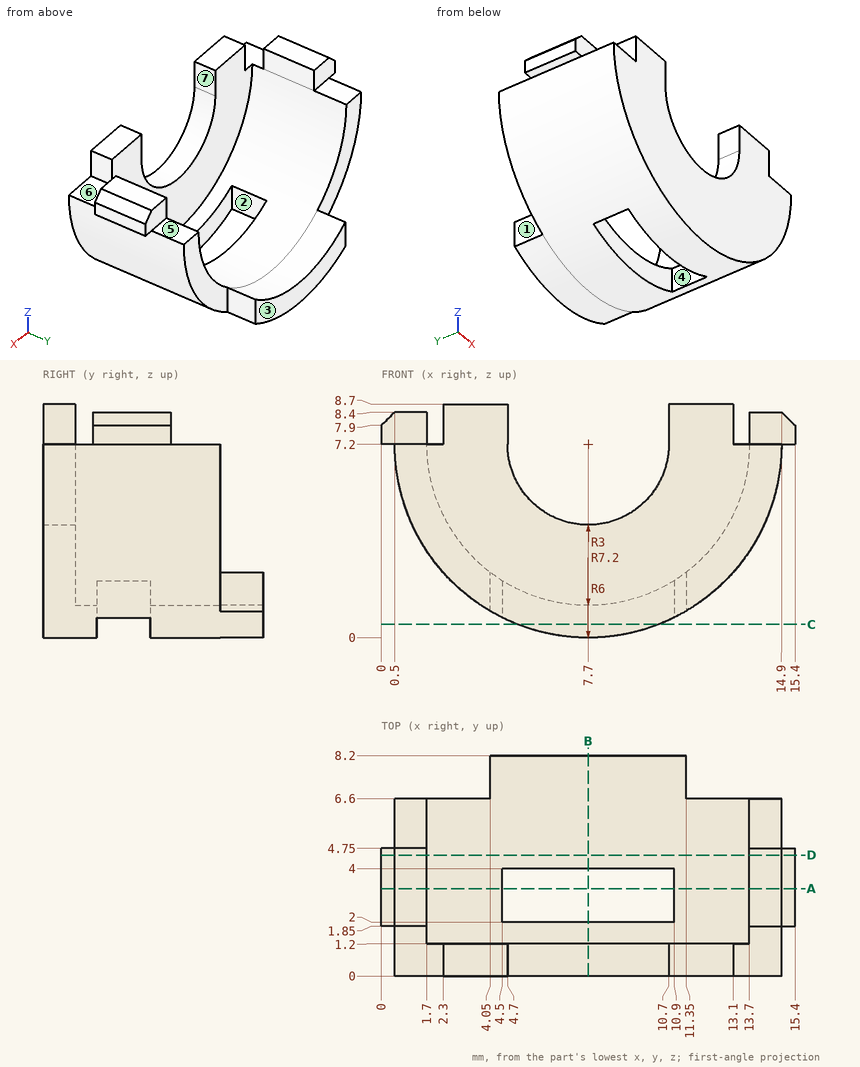
Geometry check sheet. Reference: drawing and pictorial views, mm from the part's lowest x, y, z. A direction names the side the tool comes from. Round coordinates to 2 decimals unless told otherwise and drop trailing zeros. Loops run counter-clockwise (first coordinate to the right, second up) from the corner with the lowest first, then second, coordinate; pieces in that order, holes last. Notation, with made-up numbers: M -37,6.5 L -31,6.5 A28 cw -31,36.5 Z; hole C 0.5,-1 d10. An arc over 180 degrees is marked long. One line per item, written item: value.
(1) Sectioned sample at B-B, the plane x = 7.7. Record the cut outline in (y, z), then the cut area to 3 significant figures.
Computed values:
outline: M 0,0 L 2,0 L 2,1.2 L 1.2,1.2 L 1.2,4.2 L 0,4.2 Z; M 4,0 L 8.2,0 L 8.2,1.2 L 4,1.2 Z
area: 11.0 mm^2
(2) Depth check by flat-ended pin: pin 1 Ø0.6 at (x, z) = (14.5, 8) entering from -Y; pin 2 Ø1 at (x, z) = (11, 3) entering from -Y; pin 3 Ø1 at (y, z) = (0.5, 7.5) entering from +X; pin 4 Ø4 at (y, z) = (7, 2) entering from +X. Enter the tip coordinate at first touch or a pass-through.
Computed values:
pin 1: stops at y = 1.85
pin 2: stops at y = 0
pin 3: stops at x = 14.9
pin 4: stops at x = 14.13
(3) Sectioned sample at A-A, the plane y = 3.25. Record the cut outline in (x, z).
Computed values:
outline: M 0,7.2 L 0.5,7.2 A7.2 ccw 4.5,0.75 L 4.5,2.12 A6 cw 1.7,7.2 L 1.7,8.4 L 0.5,8.4 L 0,7.9 Z; M 10.9,0.75 A7.2 ccw 14.9,7.2 L 15.4,7.2 L 15.4,7.9 L 14.9,8.4 L 13.7,8.4 L 13.7,7.2 A6 cw 10.9,2.12 Z
(4) Sectioned sample at D-D, the plane y = 4.5. Record the cut outline in (x, z).
Computed values:
outline: M 0,7.2 L 0.5,7.2 A7.2 ccw 14.9,7.2 L 15.4,7.2 L 15.4,7.9 L 14.9,8.4 L 13.7,8.4 L 13.7,7.2 A6 cw 1.7,7.2 L 1.7,8.4 L 0.5,8.4 L 0,7.9 Z
(5) Release check for a two-part mould opening along X. For the marked faces 1, 2 and 3 record: +X half, -X half, draft (parallel to the pull), parting line (faces both ways), or undercut.
Computed values:
face 1: -X half
face 2: undercut
face 3: draft
(6) Sectioned sample at C-C, the plane z = 0.5. Record the cut outline in (x, y), then the cut area to 3 significant figures.
Computed values:
outline: M 5.06,0 L 10.34,0 L 10.34,2 L 5.06,2 Z; M 5.06,4 L 10.34,4 L 10.34,8.2 L 5.06,8.2 Z
area: 32.7 mm^2
(7) Thickness scan on line 1 (X direction, y = 3.25, z = 7.5); line 2 (X direction, y = 6.5, z = 7); line 3 (Y direction, x = 6.5, z = 1). Record the ranges inside material, lowest first.
Computed values:
line 1: x = 0 to 1.7, 13.7 to 15.4
line 2: x = 0.5 to 1.7, 13.7 to 14.9
line 3: y = 0 to 2, 4 to 8.2
(8) Access from +Z, -Z, +X, -X, +Y, -Y to the whole of each face (thin tool, end or side, straight path). Record for the marked faces 4, 5, 6 and 7.
Computed values:
face 4: +Z, -Z
face 5: +Z, +X, -X, +Y
face 6: +Z, +X, -Y
face 7: +Z, +Y, -Y
